Check sheet for the drawn part. Datum: minimum x, y, z corner. Units: mm. Round coordinates to 2 decimals unless told otherwise and drop trailing zeros. Loops run counter-clockwise (first coordinate to the right, second up) from the corner with the lowest first, then second, coordinate; pieces in that order, holes last.
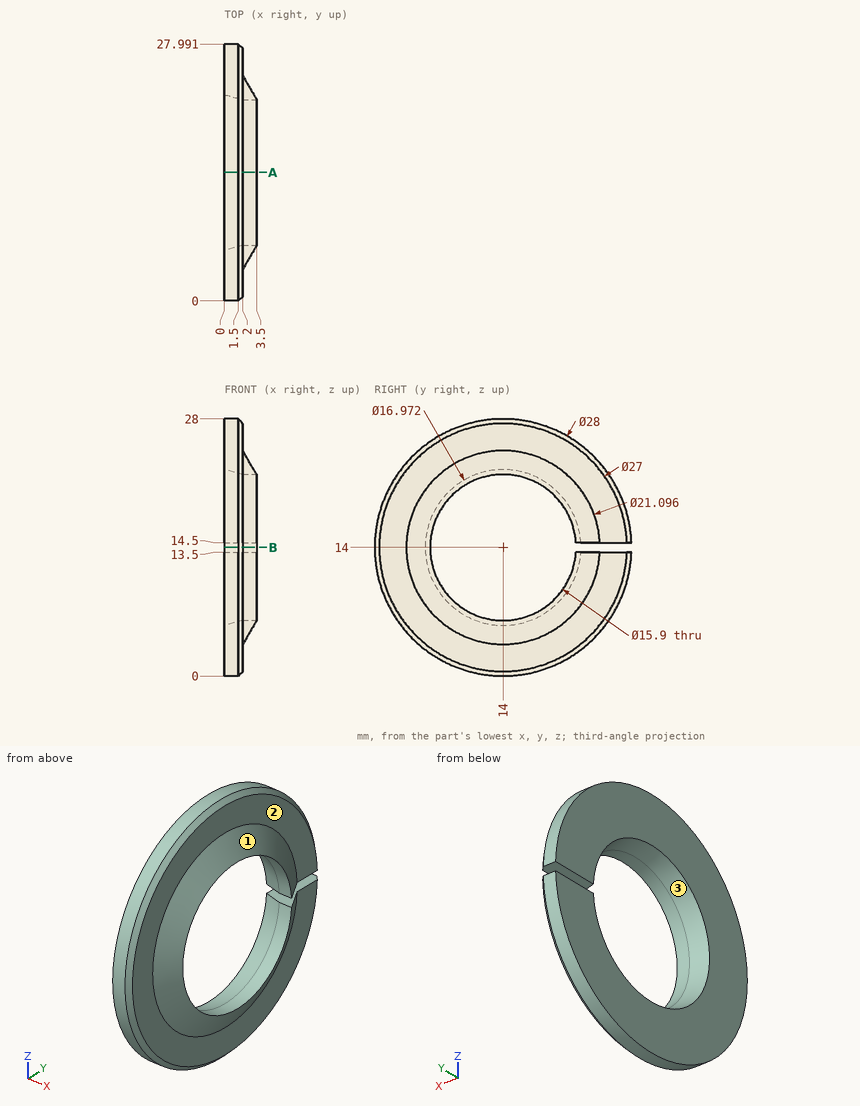
1) Mould release check, pull along Z, two halves, no side actions. Record for the marked faces 1, 2 and 3: +Z half, -Z half, draft (parallel to the pull), parting line (faces both ways), or undercut.
Report:
face 1: parting line
face 2: draft
face 3: undercut
2) Scan lines: line 1 along X through (y, z) = (11, 1.25); line 2 along Y through (x, z) = (0.65, 8.75); line 3 along Y through (x, z) = (1.35, 19). Record each from-to range of solid material in increasing order.
Report:
line 1: x = 0 to 2
line 2: y = 1.02 to 7.56, 20.44 to 26.98
line 3: y = 0.92 to 7.6, 20.4 to 27.08
3) Gauge pin test, flat ends, axial feed: pin 1 (5 mm diameter, centred on y = 16.5, z = 8.5, fed in from -X); pin 2 (1.8 mm diameter, centred on x = 1.5, y = 25.5, fed in from +Z) (1 decimal); pin 3 (1 mm diameter, centred on x = 1, z = 9, fed in from -Y); pin 4 (1 mm diameter, centred on x = 1.5, y = 17, fed in from -Z) (3 decimals). Record the tip position at first contact, or that the pin passes through.
Report:
pin 1: stops at x = 0
pin 2: stops at z = 23.1
pin 3: stops at y = 0.74
pin 4: stops at z = 0.225
4) Sectioned sample at A-A, the plane y = 14. Record the cut outline in (x, z).
Report:
outline: (0, 0) - (1.5, 0) - (2, 0.5) - (2, 3.45) - (3.5, 6.05) - (2, 6.05) - (0, 5.51) - close; (0, 22.49) - (2, 21.95) - (3.5, 21.95) - (2, 24.55) - (2, 27.5) - (1.5, 28) - (0, 28) - close
5) Sectioned sample at B-B, the plane z = 14. Record the cut outline in (x, y).
Report:
outline: (0, 0) - (1.5, 0) - (2, 0.5) - (2, 3.45) - (3.5, 6.05) - (2, 6.05) - (0, 5.51) - close
